```python
from build123d import *

# Parameters (mm, degrees)
SKETCH007_R     = 2.1
PAD003_DEPTH    = 10
SKETCH_R        = 16
PAD_DEPTH       = 3
POCKET_DEPTH    = 3.001
POCKET001_DEPTH = 3
POCKET002_DEPTH = 3
SKETCH004_R     = 6
PAD001_DEPTH    = 6
SKETCH005_R     = 3.5
PAD002_DEPTH    = 2
SKETCH006_R     = 2.1
POCKET003_DEPTH = 11.001
FILLET_R        = 1.5
FILLET001_R     = 0.8


with BuildPart() as pad003:
    # Sketch007 → Pad003 (new body)
    with BuildSketch(Plane.XZ):
        with Locations((0, 6)):
            Circle(SKETCH007_R)
    extrude(amount=PAD003_DEPTH)


with BuildPart() as cut:
    # Sketch → Pad (new body)
    with BuildSketch(Plane.XY):
        Circle(SKETCH_R)
    extrude(amount=PAD_DEPTH)

    # Sketch001 → Pocket (cut, through all)
    with BuildSketch(Plane.XY.offset(3)):
        with BuildLine():
            ThreePointArc((-2.847664, -14.048884), (9.073595, -11.097307), (14.334585, 0))
            ThreePointArc((14.334585, 0), (12.334585, 2), (10.334585, 0))
            ThreePointArc((-2.053037, -10.128608), (6.54165, -8.000654), (10.334585, 0))
            ThreePointArc((-2.053037, -10.128608), (-4.410489, -11.691432), (-2.847664, -14.048884))
        make_face()
    extrude(amount=-POCKET_DEPTH, mode=Mode.SUBTRACT)

    # Sketch002 → Pocket001 (cut)
    with BuildSketch(Plane.XY.offset(3)):
        with BuildLine():
            ThreePointArc((-10.443847, 1.041795), (-10.47921, -0.587733), (-10.261856, -2.203087))
            ThreePointArc((-14.172744, -3.042704), (-11.797491, -4.57834), (-10.261856, -2.203087))
            ThreePointArc((-14.424094, 1.438832), (-14.472934, -0.811724), (-14.172744, -3.042704))
            ThreePointArc((-10.443847, 1.041795), (-12.235452, 3.230437), (-14.424094, 1.438832))
        make_face()
    extrude(amount=-POCKET001_DEPTH, mode=Mode.SUBTRACT)

    # Sketch003 → Pocket002 (cut)
    with BuildSketch(Plane.XY.offset(3)):
        with BuildLine():
            ThreePointArc((-8.510484, 11.534817), (-9.061837, 11.106909), (-9.59171, 10.652673))
            ThreePointArc((-9.59171, 10.652673), (-9.739738, 7.828122), (-6.915187, 7.680094))
            ThreePointArc((-6.135673, 8.316079), (-6.533173, 8.007578), (-6.915187, 7.680094))
            ThreePointArc((-6.135673, 8.316079), (-5.71371, 11.112854), (-8.510484, 11.534817))
        make_face()
    extrude(amount=-POCKET002_DEPTH, mode=Mode.SUBTRACT)

    # Sketch004 → Pad001 (new body)
    with BuildSketch(Plane.XY.offset(3)):
        Circle(SKETCH004_R)
    extrude(amount=PAD001_DEPTH)

    # Sketch005 → Pad002 (new body)
    with BuildSketch(Plane.XY.offset(9)):
        Circle(SKETCH005_R)
    extrude(amount=PAD002_DEPTH)

    # Sketch006 → Pocket003 (cut, through all)
    with BuildSketch(Plane.XY.offset(11)):
        Circle(SKETCH006_R)
    extrude(amount=-POCKET003_DEPTH, mode=Mode.SUBTRACT)

    # Fillet
    fillet_edges = [cut.edges().sort_by_distance(p)[0] for p in [
        (-3.5, 0, 9),
    ]]
    fillet(fillet_edges, radius=FILLET_R)

    # Fillet001
    fillet001_edges = [cut.edges().sort_by_distance(p)[0] for p in [
        (-6, 0, 9),
    ]]
    fillet(fillet001_edges, radius=FILLET001_R)

    # Cut: cut Pad003
    add(pad003.part, mode=Mode.SUBTRACT)


solid = cut.part
```
Geometry: final body of the model. Coordinates: model frame, mm. A direction names the side the tool comes from. Round coordinates to 2 decimals unless told otherwise and drop trailing zeros. Write each loop counter-clockwise with the first axis right and the second up, starting at its lowest first coordinate (ties: lowest second). Pieces come first, ordered by that corner, then holes.
Item 1: Section query A-A (x = 0). Return loops of the section in (y, z).
Item 2: Section query B-B (x = -11). Return loops of the section in (y, z), plus the area to 3 significant figures.
Item 3: Section query D-D (y = -4). Give the number of separate pieces and of enclosed holes in the cut face, plus the area to 3 significant figures.
Item 4: Set-up query: faces 1 (the face through (0, 7, 3)), 2 (the face through (2.003, -3.626, 6.631)), 3 (the face through (-10.48, -0.56, 1.52)). Return all of +Z, -Z, +X, -X, +Y, -Y with unobstructed straight access to the full face (end or side cutting, diameter ignored); none if empty.
Item 5: Material intervals for L1, parallel to X at y = -1, z = 2.5; L2, parallel to Y at x = -1, z = 1; L3, parallel to Z at x = 1, y = -5, sorted ascending.
Item 6: Pin query (flat end, axial travel): P1, Ø8, axis at x = 8.5, y = -9.5, coming from the -Z side; P2, Ø5, axis at x = 12, z = 1.5, coming from the -Y side; P3, Ø5.5, axis at x = 0, z = 6, coming from the -Y side; P4, Ø2, axis at x = -6.5, y = 2, coming from the +Z side. Return the tip coordinate at first contact, or that it passes through.
Item 7: Mould query, pull axis X, two halves, no side actions, for faces 4 (the face through (-14.475, -0.78, 1.521)), 5 (the face through (3.233, -1.341, 10.746)), 6 (the face through (0, 4, 0)), 7 (the face through (-5.69, 11.08, 1.52)). Classes: +X half, -X half, draft (parallel to the pull), parting line (faces both ways), or undercut.
Item 8: Section query C-C (z = 1). Return loops of the section in (x, y).
Completed:
1. outline: (-16, 0) - (-14.33, 0) - (-14.33, 3) - (-16, 3) - close; (-10.33, 0) - (-2.1, 0) - (-2.1, 3.9) - (-6, 3.9) - (-6, 3) - (-10.33, 3) - close; (-6, 8.1) - (-2.1, 8.1) - (-2.1, 11) - (-3.5, 11) - (-3.5, 10.5) arc R1.5 cw to (-5, 9) - (-5.2, 9) arc R0.8 ccw to (-6, 8.2) - close; (2.1, 0) - (16, 0) - (16, 3) - (6, 3) - (6, 8.2) arc R0.8 ccw to (5.2, 9) - (5, 9) arc R1.5 cw to (3.5, 10.5) - (3.5, 11) - (2.1, 11) - close
2. outline: (-11.62, 0) - (-4.21, 0) - (-4.21, 3) - (-11.62, 3) - close; (2.63, 0) - (11.62, 0) - (11.62, 3) - (2.63, 3) - close
2. area: 49.2 mm2
3. separate pieces: 3
3. enclosed holes: 1
3. area: 112 mm2
4. face 1: +Z
4. face 2: -Y
4. face 3: +Z, -Z
5. L1: x = -15.97 to -14.46, -10.45 to -1.85, 1.85 to 10.29, 14.3 to 15.97
5. L2: y = -15.97 to -14.3, -10.29 to -1.85, 1.85 to 15.97
5. L3: z = 0 to 4.15, 7.85 to 9
6. P1: stops at z = 0
6. P2: stops at y = -12.87
6. P3: stops at y = -6
6. P4: stops at z = 8.73
7. face 4: undercut
7. face 5: parting line
7. face 6: draft
7. face 7: undercut
8. outline: circle Ø32 at (0, 0); hole (-14.42, 1.44) arc R14.5 ccw to (-14.17, -3.04) arc R2 ccw to (-10.26, -2.2) arc R10.5 cw to (-10.44, 1.04) arc R2 ccw to start; hole (-9.59, 10.65) arc R2 ccw to (-6.92, 7.68) arc R10.33 cw to (-6.14, 8.32) arc R2 ccw to (-8.51, 11.53) arc R14.34 ccw to start; hole (-2.85, -14.05) arc R14.33 ccw to (14.33, 0) arc R2 ccw to (10.33, 0) arc R10.33 cw to (-2.05, -10.13) arc R2 ccw to start; hole circle Ø4.2 at (0, 0)
